from build123d import *

# Parameters (mm, degrees)
BOSS_EXTRUDE1_DEPTH = 25.4
CUT_EXTRUDE1_DEPTH  = 2217.171715999
SWEEP2_PROFILE_R    = 12.7


with BuildPart() as part:
    # Sketch1 → Boss-Extrude1 (new body)
    with BuildSketch(Plane.XY):
        with BuildLine():
            Line((-318.401962341, 0), (873.874037659, 0))
            Line((873.874037659, 0), (873.874037659, 1883.156))
            ThreePointArc((873.874037659, 1883.156), (829.553846601, 1991.493828188), (721.476635331, 2036.44581097))
            Line((721.476635331, 2036.44581097), (390.514635331, 2036.44581097))
            ThreePointArc((390.514635331, 2036.44581097), (-68.281974684, 1851.0799482), (-269.546688357, 1399.032))
            Line((-269.546688357, 1399.032), (-318.401962341, 0))
        make_face()
        with BuildLine():
            Line((-156.242870874, 1004.607855187), (-142.624053326, 1394.599763919))
            ThreePointArc((-142.624053326, 1394.599763919), (19.939638364, 1759.723793557), (390.514635331, 1909.44581097))
            Line((390.514635331, 1909.44581097), (721.476635331, 1909.44581097))
            ThreePointArc((721.476635331, 1909.44581097), (739.565122057, 1901.8774303), (746.874037659, 1883.682554903))
            Line((746.874037659, 1883.682554903), (746.874037659, 1005.341277451))
            Line((746.874037659, 1005.341277451), (-156.242870874, 1004.607855187))
        make_face(mode=Mode.SUBTRACT)
    extrude(amount=BOSS_EXTRUDE1_DEPTH)

    # Sketch2 → Cut-Extrude1 (cut, through all)
    with BuildSketch(Plane.XY.offset(25.4)):
        Polygon((873.874037659, 1232.505665346), (873.874037659, 1283.305665346), (848.474037659, 1283.305665346), (848.474037659, 1181.705665346), (873.874037659, 1181.705665346), align=None)
        Polygon((873.874037659, 523.771597211), (873.874037659, 574.571597211), (848.474037659, 574.571597211), (848.474037659, 472.971597211), (873.874037659, 472.971597211), align=None)
    extrude(amount=-CUT_EXTRUDE1_DEPTH, mode=Mode.SUBTRACT)

    # Sweep2: sweep along a path in Sketch5
    with BuildLine(Plane(origin=(0, 889, 0), x_dir=(1, 0, 0), z_dir=(0, 1, 0))) as sweep2_path:
        Line((-156.242870874, -25.4), (-156.242870874, -76.2))
        Line((-156.242870874, -76.2), (60.483973487, -76.2))
        Line((60.483973487, -76.2), (60.483973487, -25.4))
        Line((60.483973487, -25.4), (60.483973487, 0))
        Line((60.483973487, 0), (60.483973487, 50.8))
        Line((60.483973487, 50.8), (-156.242870874, 50.8))
        Line((-156.242870874, 50.8), (-156.242870874, 0))
    # Sweep2 profile (on start of the path) → Sweep2 (sweep)
    with BuildSketch(Plane(origin=(-156.242870874, 889, 25.4), x_dir=(1, 0, 0), z_dir=(0, 0, 1))):
        Circle(SWEEP2_PROFILE_R)
    sweep(path=sweep2_path.line, transition=Transition.RIGHT)


solid = part.part
Verification items for the finished model (mm, model axes). Give positions to 0.01 mm unless a question says otherwise; leave off trailing zeros. Write each loop counter-clockwise with the first axis right and the second up, starting at its lowest first coordinate (ties: lowest second). Pieces come first, ordered by that corner, then holes. Notation, with made-up numbers: M 51,72 L 91,72 A16 cw 91,100 Z; hole C 24.25,58 d2. An arc over 180 degrees is marked long. Put each result on its own line as item: value. Start each with the question number.
1. Draft check along X on faces 1 (the face through (830.733, 1990.295, 12.522)), 2 (the face through (-63.148, 1855.985, 12.522)), 3 (the face through (15.84, 1755.72, 12.52)). Enter one of: +X half, -X half, draft (parallel to the pull), parting line (faces both ways), or undercut.
2. Go/stop test with flat-tipped pins: pin 1 Ø7.5 at (y, z) = (1575, 16.5) entering from +X; pin 2 Ø20.5 at (y, z) = (505, 15) entering from +X; pin 3 Ø20.5 at (y, z) = (1468, 13) entering from -X. Record where each tip stops, or that it passes through.
3. Section check C-C (x = 441). Record the cut outline in (y, z), and give its area (3 significant figures).
4. Scan lines: line 1 along Y through (x, z) = (539.5, 18); line 2 along Y through (x, z) = (684, 2); line 3 along Z through (x, y) = (-181.5, 352.5). Record each from-to range of solid material in increasing order. Write a range as [from, to].
5. Section check A-A (x = 21.5). Record the cut outline in (y, z), and give its area (3 significant figures).
6. Section check B-B (y = 1651). Record the cut outline in (x, z).
Answer list:
1. face 1: +X half
1. face 2: -X half
1. face 3: undercut
2. pin 1: x = 873.87
2. pin 2: x = 848.47
2. pin 3: x = -264.87
3. outline: M 0,0 L 1005.09,0 L 1005.09,25.4 L 0,25.4 Z; M 1909.45,0 L 2036.45,0 L 2036.45,25.4 L 1909.45,25.4 Z
3. area: 28,800 mm2
4. line 1: [0, 1005.17], [1909.45, 2036.45]
4. line 2: [0, 1005.29], [1909.45, 2036.45]
4. line 3: [0, 25.4]
5. outline: M 0,0 L 1004.75,0 L 1004.75,25.4 L 0,25.4 Z; C 889,-50.8 d25.4; C 889,76.2 d25.4; M 1761.22,0 L 1923.74,0 L 1923.74,25.4 L 1761.22,25.4 Z
5. area: 30,700 mm2
6. outline: M -209.97,0 L -66.59,0 L -66.59,25.4 L -209.97,25.4 Z; M 746.87,0 L 873.87,0 L 873.87,25.4 L 746.87,25.4 Z
